Verification items for this drawing (mm, ordinates from the low corner). A direction names the side the tool comes from. Round coordinates to 2 decimals unless told otherwise and drop trailing zeros. Order: outer loops, then holes, each group sorted by start corner. A loop starts at its lowest first (then second) coordinate and runs counter-clockwise, first axis right, second up. Notation, with made-up numbers: (58.5, -20.5) - (72.5, -20.5) arc R15 ccw to (72.5, -2.5) - close; hole circle Ø9 at (-22, -17.75). An arc over 180 degrees is marked (long way). Use a Markdown table: item, result. Add a question column.
(1) Section check D-D on z = 11.5. Record the boundary of the cut face in (x, y).
(2) Mould release check, pull along X, two halves, no side actions. Record for the marked faces 1, 2, 3 and 4: released by +X, released by -X, zero draft, split by the parting line, or undercut.
(3) Section check A-A on y = 25. Record the boundary of the cut face in (x, z), then the cut area to 3 significant figures.
(4) Thickness scan on line 1 along Y through (x, z) = (20, 0.4); line 2 along Y through (x, z) = (24.6, 5); line 3 along X through (y, z) = (75, 24.75). Record the ranges inside material, lowest first. Write a range as [from, to].
(5) Gauge pin test, flat end, axial feed: P1, Ø5, axis at x = 6, z = 3.5, coming from the +Y side. Record the tip position at first contact, or that the pin passes through.
(6) Section check B-B on x = 13.25. Record the boundary of the cut face in (y, z), then the cut area to 3 significant figures.
(7) Section check C-C on z = 20. Give the number of separate pieces and of enclosed holes in the cut face, then the cut area to 3 significant figures.
(8) Access from +Z, -Z, +X, -X, +Y, -Y to the whole of each face (thin tool, end or side, straight path). Record for the marked faces 5 and 6.
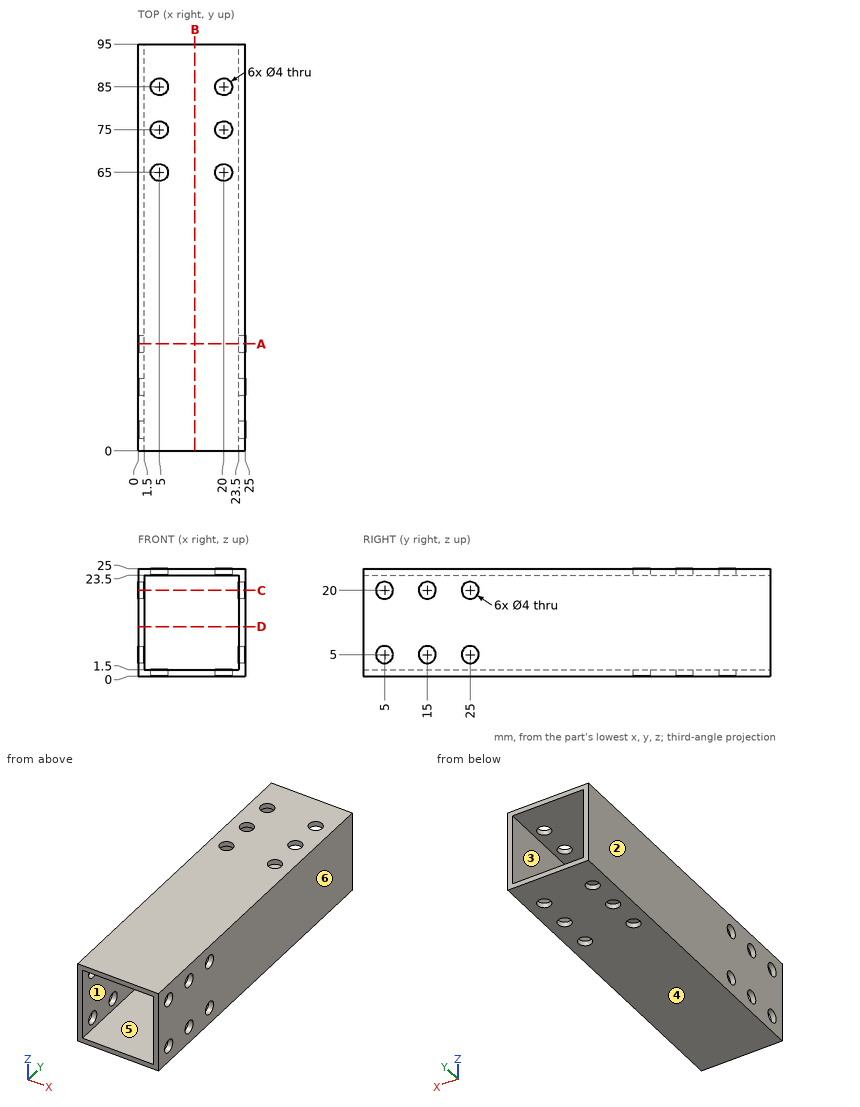
Check sheet entries:
| question | item | result |
|---|---|---|
| 1 | outline | (0, 0) - (1.5, 0) - (1.5, 95) - (0, 95) - close; (23.5, 0) - (25, 0) - (25, 95) - (23.5, 95) - close |
| 2 | face 1 | undercut |
| 2 | face 2 | released by -X |
| 2 | face 3 | undercut |
| 2 | face 4 | zero draft |
| 3 | outline | (0, 0) - (25, 0) - (25, 3) - (23.5, 3) - (23.5, 1.5) - (1.5, 1.5) - (1.5, 3) - (0, 3) - close; (0, 7) - (1.5, 7) - (1.5, 18) - (0, 18) - close; (0, 22) - (1.5, 22) - (1.5, 23.5) - (23.5, 23.5) - (23.5, 22) - (25, 22) - (25, 25) - (0, 25) - close; (23.5, 7) - (25, 7) - (25, 18) - (23.5, 18) - close |
| 3 | area | 117 mm2 |
| 4 | line 1 | y = [0, 63], [67, 73], [77, 83], [87, 95] |
| 4 | line 2 | y = [0, 3], [7, 13], [17, 23], [27, 95] |
| 4 | line 3 | x = [0, 3], [7, 18], [22, 25] |
| 5 | P1 | stops at y = 95 |
| 6 | outline | (0, 0) - (95, 0) - (95, 1.5) - (0, 1.5) - close; (0, 23.5) - (95, 23.5) - (95, 25) - (0, 25) - close |
| 6 | area | 285 mm2 |
| 7 | separate pieces | 8 |
| 7 | enclosed holes | 0 |
| 7 | area | 249 mm2 |
| 8 | face 5 | +Y, -Y |
| 8 | face 6 | +Z, -Z, +X, +Y, -Y |
